from build123d import *

# Parameters (mm, degrees)
SCALE1_SCALE = 1.5


with BuildPart() as part:
    # Sketch1 → Revolve1 (revolve)
    with BuildSketch(Plane.XY, mode=Mode.PRIVATE) as revolve1_sk:
        with BuildLine():
            Line((12.7, 12.80502263), (12.7, 101.6))
            Line((12.7, 101.6), (25.399381994, 101.6))
            Line((25.399381994, 101.6), (25.399381994, 111.76))
            ThreePointArc((25.399381994, 111.76), (51.978144098, 155.533163358), (28.151294552, 200.863083566))
            Line((28.151294552, 200.863083566), (-0.000618006, 200.863083566))
            Line((-0.000618006, 200.863083566), (-28.152530564, 200.863083566))
            ThreePointArc((-28.152530564, 200.863083566), (-51.97938011, 155.533163358), (-25.400618006, 111.76))
            Line((-25.400618006, 111.76), (-25.400618006, 101.6))
            Line((-25.400618006, 101.6), (-12.7, 101.6))
            Line((-12.7, 101.6), (-12.7, 12.80502263))
            Line((-12.7, 12.80502263), (12.7, 12.80502263))
        make_face()
    revolve(revolve1_sk.sketch.rotate(Axis((12.7, 0, 0), (-1, 0, 0)), 90), axis=Axis((12.7, 0, 0), (-1, 0, 0)))


with BuildPart() as part_1:
    # Scale1: scaled about (-0.000562241, 0, 0)
    add(part.part.scale(SCALE1_SCALE).moved(Location((0.00028112, 0, 0))))


solid = part_1.part
Read the model definition and answer for the solid it produces. Units are mm, in the model's axes. A direction names the side the tool comes from. Coordinates: 2 decimals unless noted, no trailing zeros. Write each loop counter-clockwise with the first axis right and the second up, starting at its lowest first coordinate (ties: lowest second). Pieces come first, ordered by that corner, then holes. Notation, with made-up numbers: (-28.5, -17.75) - (-1.5, -17.75) arc R19 cw to (-1.5, -13.75) - close; hole circle Ø8 at (80, -18.75). An arc over 180 degrees is marked (long way). One line per question, with ' | ' between items.
Q1. Consider L1, parallel to Y at x = 34, z = 0; L2, parallel to Y at x = 6, z = 0; L3, parallel to Z at x = 34.5, y = 4. Determine where each line is inside the solid, lowest interval first. Write a range as [from, to].
Result set:
L1: [-301.29, -152.4], [152.4, 301.29] | L2: [-301.29, -19.21], [19.21, 301.29] | L3: [-301.27, -152.35], [152.35, 301.27]
Q2. Find section A-A, the plane z = 0. Write down the section's boundary in (x, y).
Result set:
outline: (-42.23, -301.29) - (42.23, -301.29) arc R78.01 ccw to (38.1, -167.64) - (38.1, -152.4) - (19.05, -152.4) - (19.05, -19.21) - (-19.05, -19.21) - (-19.05, -152.4) - (-38.1, -152.4) - (-38.1, -167.64) arc R78.01 ccw to start; (-42.23, 301.29) arc R78.01 ccw to (-38.1, 167.64) - (-38.1, 152.4) - (-19.05, 152.4) - (-19.05, 19.21) - (19.05, 19.21) - (19.05, 152.4) - (38.1, 152.4) - (38.1, 167.64) arc R78.01 ccw to (42.23, 301.29) - close
Q3. Find section C-C, the plane x = 2. Write down the section's boundary in (y, z), plus the area to 3 significant figures.
Result set:
outline: circle Ø602.59 at (0, 0); hole circle Ø38.42 at (0, 0) | area: 284,000 mm^2
Q4. Each of these flat-tipped pins is pushed along its axis until it touches: P1, Ø6, axis at y = -225.5, z = -176.5, coming from the -X side; P2, Ø6, axis at x = -42.5, y = -238.5, coming from the +Z side; P3, Ø8, axis at x = -30.5, y = 115.5, coming from the +Z side. Where does it stop, or does it pass through?
Result set:
P1: x = -61.76 | P2: z = 187.92 | P3: z = 279.9
Q5. For faces 3 (the cylindrical face through (0.27, -5.77, -18.32)), 4 (the cylindrical face through (28.71, 92.73, 120.94)), 5 (the flat face through (-38.101, 148.2, -36.5)), determine the directions among +Z, -Z, +X, -X, +Y, -Y from which every point of the face is accessible in a straight line to the end or side of a thin tool.
Result set:
face 3: +X, -X | face 4: +X | face 5: -X
Q6. Determine the mould class of faces 1 (the cylindrical face through (-0.592, -13.247, 301.003)), 2 (the flat face through (38.099, 148.2, 36.5)) for opening direction Y: +Y half, -Y half, draft (parallel to the pull), parting line (faces both ways), or undercut.
Result set:
face 1: parting line | face 2: undercut
